The listing builds one solid part. Answer for the finished solid, in the listing's coordinates (mm). Face numbers are marked on the shaded views. A direction names the side the tool comes from. Coordinates: 2 decimals unless noted, no trailing zeros. Write each loop counter-clockwise with the first axis right and the second up, starting at its lowest first coordinate (ties: lowest second). Pieces come first, ordered by that corner, then holes. Notation, with made-up numbers: M -20.75,79 L 3.25,79 A27 ccw 3.25,107 Z; hole C 78,21.5 d4. An arc over 180 degrees is marked long. Answer as CSV lines item,"result".
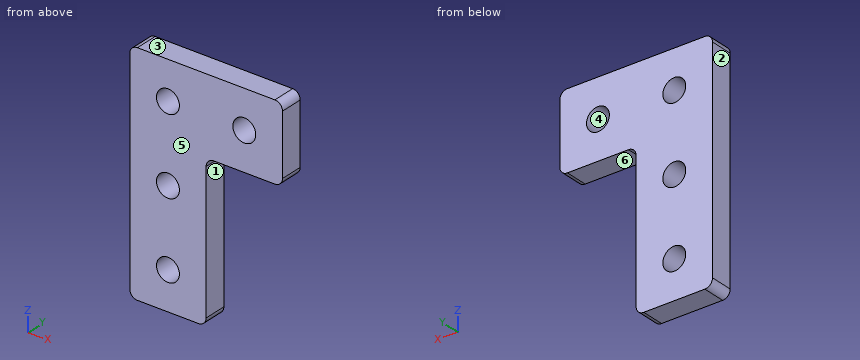
```python
from build123d import *

# Parameters (mm, degrees)
SKETCH1_R           = 1.5
BOSS_EXTRUDE1_DEPTH = 3
FILLET1_R           = 1
FILLET2_R           = 1


with BuildPart() as part:
    # Sketch1 → Boss-Extrude1 (new body)
    with BuildSketch(Plane(origin=(0, 0, 0), x_dir=(1, 0, 0), z_dir=(0, 1, 0))):
        Polygon((0, 0), (10, 0), (20, 0), (20, 10), (10, 10), (10, 30), (0, 30), align=None)
        with Locations((5, 25)):
            Circle(SKETCH1_R, mode=Mode.SUBTRACT)
        with Locations((5, 15)):
            Circle(SKETCH1_R, mode=Mode.SUBTRACT)
        with Locations((5, 5)):
            Circle(SKETCH1_R, mode=Mode.SUBTRACT)
        with Locations((15, 5)):
            Circle(SKETCH1_R, mode=Mode.SUBTRACT)
    extrude(amount=BOSS_EXTRUDE1_DEPTH)

    # Fillet1
    fillet1_edges = [part.edges().sort_by_distance(p)[0] for p in [
        (10, 1.5, -10),
    ]]
    fillet(fillet1_edges, radius=FILLET1_R)

    # Fillet2
    fillet2_edges = [part.edges().sort_by_distance(p)[0] for p in [
        (0, 1.5, -30),
        (10, 1.5, -30),
        (20, 1.5, -10),
        (20, 1.5, 0),
        (0, 1.5, 0),
    ]]
    fillet(fillet2_edges, radius=FILLET2_R)


solid = part.part
```
Q1. The mould has two halves that part along Z. Classify the marked faces 3, 4, 5 and 6: pulls with the +Z half, pulls with the -Z half, needs draft (parallel to the pull), parting line crosses it, or undercut.
Output:
face 3,"pulls with the +Z half"
face 4,"undercut"
face 5,"needs draft"
face 6,"pulls with the -Z half"
Q2. Find section D-D (y = 1.7). Give the vertices of the cut face in (x, z).
Output:
outline,"M 0,-29 A1 ccw 1,-30 L 9,-30 A1 ccw 10,-29 L 10,-11 A1 cw 11,-10 L 19,-10 A1 ccw 20,-9 L 20,-1 A1 ccw 19,0 L 1,0 A1 ccw 0,-1 Z; hole C 5,-25 d3; hole C 5,-15 d3; hole C 5,-5 d3; hole C 15,-5 d3"
Q3. Find section A-A (z = -5). Give the vertices of the cut face in (x, y).
Output:
outline,"M 0,0 L 3.5,0 L 3.5,3 L 0,3 Z; M 6.5,0 L 13.5,0 L 13.5,3 L 6.5,3 Z; M 16.5,0 L 20,0 L 20,3 L 16.5,3 Z"
Q4. For the marked faces 1 and 2, determine the directions among +Z, -Z, +X, -X, +Y, -Y from which every point of the face is accessible in a straight line to the end or side of a thin tool.
Output:
face 1,"-Z, +X, +Y, -Y"
face 2,"+Z, -Z, -X, +Y, -Y"
Q5. Find section C-C (x = 15). Give the vertices of the cut face in (y, z), and give its area (3 significant figures).
Output:
outline,"M 0,-10 L 3,-10 L 3,-6.5 L 0,-6.5 Z; M 0,-3.5 L 3,-3.5 L 3,0 L 0,0 Z"
area,"21.0 mm2"
Q6. Straight lines are drawn through the part: line 1 (Z direction, x = 5, y = 1.4); line 2 (X direction, y = 1.55, z = -5); line 3 (Z direction, x = 5.5, y = 2.5). For each, find the intervals that lie inside material, in ascending order.
Output:
line 1,"-30 to -26.5, -23.5 to -16.5, -13.5 to -6.5, -3.5 to 0"
line 2,"0 to 3.5, 6.5 to 13.5, 16.5 to 20"
line 3,"-30 to -26.41, -23.59 to -16.41, -13.59 to -6.41, -3.59 to 0"
Q7. Flat-ended cylindrical pins translate along their axes: pin 1 Ø0.9 at (y, z) = (2, -19) entering from +X; pin 2 Ø0.9 at (x, y) = (15.5, 1.5) entering from -Z. Find the tip coordinate at first contact, or state that the pin passes through.
Output:
pin 1,"x = 10"
pin 2,"z = -10"
Q8. Find section B-B (z = -15). Give the vertices of the cut face in (x, y), and give its area (3 significant figures).
Output:
outline,"M 0,0 L 3.5,0 L 3.5,3 L 0,3 Z; M 6.5,0 L 10,0 L 10,3 L 6.5,3 Z"
area,"21.0 mm2"
